Study the drawing (mm; zero at the part's minimum x, y, z) and answer. Coordinates: 2 decimals unless noted, no trailing zeros. Loops run counter-clockwise (first coordinate to the right, second up) from the corner with the lowest first, then second, coordinate; pieces in that order, holes last. Notation, with made-up numbers: (-6, 35.5) - (52, 35.5) arc R22 ccw to (52, 41.5) - close; hole circle Ø6 at (-33.75, 30.25). An arc over 180 degrees is marked (long way). Put each result on its own line as item: value.
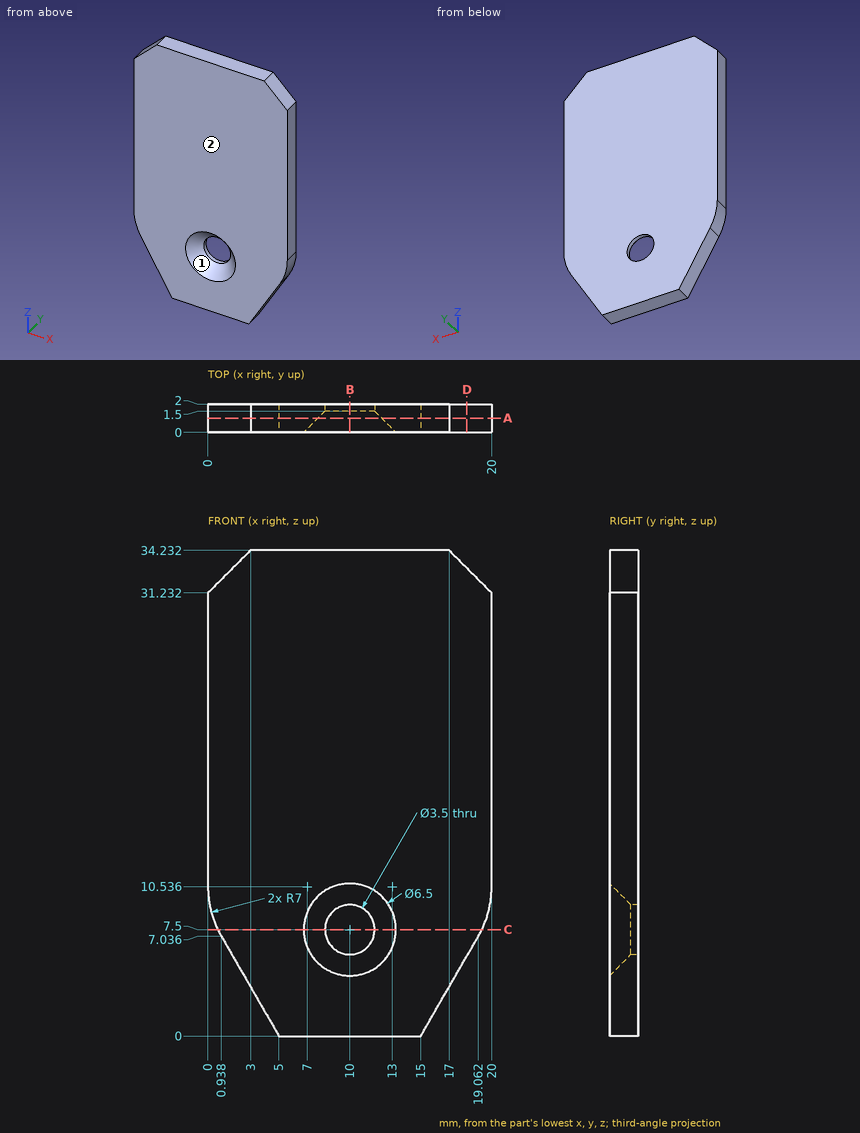
1) The part is cut by section A-A (y = 1). Give the vertices of the cut face in (x, z), and give its area (3 significant figures).
Found:
outline: (0, 10.54) arc R7 ccw to (0.94, 7.04) - (5, 0) - (15, 0) - (19.06, 7.04) arc R7 ccw to (20, 10.54) - (20, 31.23) - (17, 34.23) - (3, 34.23) - (0, 31.23) - close; hole circle Ø4.5 at (10, 7.5)
area: 616 mm^2
2) For a pull along Z with two mould halves and no side action, classify the marked faces 1 and 2 as pulls with the +Z half, pulls with the -Z half, needs draft (parallel to the pull), parting line crosses it, or undercut.
Found:
face 1: undercut
face 2: needs draft
3) The part is cut by section D-D (x = 18.25). Give the vertices of the cut face in (y, z).
Found:
outline: (0, 5.63) - (2, 5.63) - (2, 32.98) - (0, 32.98) - close
4) The part is cut by section C-C (z = 7.5). Give the vertices of the cut face in (x, y).
Found:
outline: (0.69, 0) - (6.75, 0) - (8.25, 1.5) - (8.25, 2) - (0.69, 2) - close; (11.75, 1.5) - (13.25, 0) - (19.31, 0) - (19.31, 2) - (11.75, 2) - close
5) Straight lines are drawn through the part: L1, parallel to X at y = 1.9, z = 7.5; L2, parallel to Z at x = 9.5, y = 0.9 (1 decimal); L3, parallel to Z at x = 11.5, y = 1.6. For each, find the intervals that lie inside material, in ascending order. Write a range as [from, to].
Found:
L1: x = [0.69, 8.25], [11.75, 19.31]
L2: z = [0, 5.2], [9.8, 34.2]
L3: z = [0, 6.6], [8.4, 34.23]
6) The part is cut by section B-B (x = 10). Give the vertices of the cut face in (y, z).
Found:
outline: (0, 0) - (2, 0) - (2, 5.75) - (1.5, 5.75) - (0, 4.25) - close; (0, 10.75) - (1.5, 9.25) - (2, 9.25) - (2, 34.23) - (0, 34.23) - close
